Geometry: final body of the model. Coordinates: model frame, mm. A direction names the side the tool comes from. Give positions to 0.01 mm unless a question says otherwise; leave off trailing zeros. Write each loop counter-clockwise with the first axis right and the second up, starting at its lowest first coordinate (ties: lowest second). Pieces come first, ordered by that corner, then holes. Notation, with made-up numbers: (45.25, 65.5) - (65.25, 65.5) arc R33 cw to (65.25, 95.5) - close; hole circle Ø9 at (44.25, 45.5). An arc over 180 degrees is marked (long way). Return JSON: item names as keys, results as strings.
from build123d import *

# Parameters (mm, degrees)
SKETCH_1_W          = 126
SKETCH_1_H          = 28
EXTRUDE_1_DEPTH     = 5
FILLET_1_R          = 5
FILLET_2_R          = 0.5
SKETCH_3_R          = 1.5
CUT_EXTRUDE_1_DEPTH = 10
SKETCH_4_R          = 5
EXTRUDE_2_DEPTH     = 3
EXTRUDE_3_DEPTH     = 13
SKETCH_6_R          = 1.5
CUT_EXTRUDE_2_DEPTH = 6
SKETCH_7_R          = 13
EXTRUDE_4_DEPTH     = 33
SKETCH_8_R          = 5
EXTRUDE_5_DEPTH     = 3
SKETCH_9_R          = 13
EXTRUDE_6_DEPTH     = 1
SKETCH_10_R         = 1
EXTRUDE_7_DEPTH     = 4
SKETCH_11_R         = 9
EXTRUDE_8_DEPTH     = 4
SKETCH_12_W         = 6
SKETCH_12_H         = 1.146117225
EXTRUDE_9_DEPTH     = 8
SKETCH_13_W         = 13
SKETCH_13_H         = 5
EXTRUDE_10_DEPTH    = 3.9


with BuildPart() as part:
    # 草图1 → 凸台-拉伸1 (new, symmetric)
    with BuildSketch(Plane.XY):
        Rectangle(SKETCH_1_W, SKETCH_1_H)
    extrude(amount=EXTRUDE_1_DEPTH, both=True)

    # 圆角1
    fillet_1_edges = [part.edges().sort_by_distance(p)[0] for p in [
        (63, -14, 0),
        (-63, -14, 0),
        (-63, 14, 0),
        (63, 14, 0),
    ]]
    fillet(fillet_1_edges, radius=FILLET_1_R)

    # 圆角2
    fillet_2_edges = [part.edges().sort_by_distance(p)[0] for p in [
        (0, -14, -5),
        (0, -14, 5),
        (63, 0, -5),
        (-63, 0, -5),
        (0, 14, -5),
        (61.535533906, 12.535533906, -5),
        (61.535533906, -12.535533906, -5),
        (-61.535533906, 12.535533906, -5),
        (-61.535533906, -12.535533906, -5),
        (-63, 0, 5),
        (63, 0, 5),
        (0, 14, 5),
        (61.535533906, 12.535533906, 5),
        (61.535533906, -12.535533906, 5),
        (-61.535533906, 12.535533906, 5),
        (-61.535533906, -12.535533906, 5),
    ]]
    fillet(fillet_2_edges, radius=FILLET_2_R)

    # 草图3 → 切除-拉伸1 (cut)
    with BuildSketch(Plane.XZ.offset(14)):
        with Locations(Location((-40, 0, 0), (0, 0, 270))):
            Circle(SKETCH_3_R)
        with Locations(Location((40, 0, 0), (0, 0, 90))):
            Circle(SKETCH_3_R)
    cut_extrude_1 = extrude(amount=-CUT_EXTRUDE_1_DEPTH, mode=Mode.SUBTRACT)

    # 草图4 → 凸台-拉伸2 (add)
    with BuildSketch(Plane.XY.offset(5)):
        with Locations((47.75, 0)):
            Circle(SKETCH_4_R)
    extrude_2 = extrude(amount=EXTRUDE_2_DEPTH)

    # 草图5 → 凸台-拉伸3 (add)
    with BuildSketch(Plane.XY.offset(8)):
        Polygon((47.75, -3.75277675), (51, -1.876388375), (51, 1.876388375), (47.75, 3.75277675), (44.5, 1.876388375), (44.5, -1.876388375), align=None)
    extrude_3 = extrude(amount=EXTRUDE_3_DEPTH)

    # 草图6 → 切除-拉伸2 (cut)
    with BuildSketch(Plane.XY.offset(21)):
        with Locations((47.75, 0)):
            Circle(SKETCH_6_R)
    cut_extrude_2 = extrude(amount=-CUT_EXTRUDE_2_DEPTH, mode=Mode.SUBTRACT)

    # 镜向1: 凸台-拉伸2, 凸台-拉伸3, 切除-拉伸2 across plane
    add(extrude_2.mirror(Plane(origin=(0, 0, 0), x_dir=(0, 0, 1), z_dir=(1, 0, 0))))
    add(extrude_3.mirror(Plane(origin=(0, 0, 0), x_dir=(0, 0, 1), z_dir=(1, 0, 0))))
    add(cut_extrude_2.mirror(Plane(origin=(0, 0, 0), x_dir=(0, 0, 1), z_dir=(1, 0, 0))), mode=Mode.SUBTRACT)

    # 草图7 → 凸台-拉伸4 (add)
    with BuildSketch(Plane(origin=(0, 0, -5), x_dir=(-1, 0, 0), z_dir=(0, 0, -1))):
        with Locations(Location((0, 0, 0), (0, 0, 180))):
            Circle(SKETCH_7_R)
    extrude(amount=EXTRUDE_4_DEPTH)

    # 草图8 → 凸台-拉伸5 (add)
    with BuildSketch(Plane(origin=(0, 0, -38), x_dir=(-1, 0, 0), z_dir=(0, 0, -1))):
        Circle(SKETCH_8_R)
    extrude(amount=EXTRUDE_5_DEPTH)

    # 草图9 → 凸台-拉伸6 (add)
    with BuildSketch(Plane(origin=(0, 0, -41), x_dir=(-1, 0, 0), z_dir=(0, 0, -1))):
        with Locations(Location((0, 0, 0), (0, 0, 180))):
            Circle(SKETCH_9_R)
    extrude(amount=EXTRUDE_6_DEPTH)

    # 草图10 → 凸台-拉伸7 (add)
    with BuildSketch(Plane(origin=(0, 0, -42), x_dir=(-1, 0, 0), z_dir=(0, 0, -1))):
        Circle(SKETCH_10_R)
    extrude(amount=EXTRUDE_7_DEPTH)

    # 草图11 → 凸台-拉伸8 (add)
    with BuildSketch(Plane(origin=(0, 0, -46), x_dir=(-1, 0, 0), z_dir=(0, 0, -1))):
        Circle(SKETCH_11_R)
    extrude(amount=EXTRUDE_8_DEPTH)

    # 草图12 → 凸台-拉伸9 (add)
    with BuildSketch(Plane(origin=(0, 0, -42), x_dir=(-1, 0, 0), z_dir=(0, 0, -1))):
        with Locations((0, 9.822897289)):
            Rectangle(SKETCH_12_W, SKETCH_12_H)
    extrude(amount=EXTRUDE_9_DEPTH)

    # 草图13 → 凸台-拉伸10 (add)
    with BuildSketch(Plane(origin=(0, 0, -42), x_dir=(-1, 0, 0), z_dir=(0, 0, -1))):
        with Locations((0.124599067, -8.685467679)):
            Rectangle(SKETCH_13_W, SKETCH_13_H)
    extrude(amount=EXTRUDE_10_DEPTH)

    # 镜向2: 切除-拉伸1 across plane
    add(cut_extrude_1.mirror(Plane.ZX), mode=Mode.SUBTRACT)


solid = part.part
Q1. Section query A-A, the plane x = 30. Return the cut outline in (y, z), plus the area to 3 significant figures.
Answer key:
{"outline": "(-14, -4.5) arc R0.5 ccw to (-13.5, -5) - (13.5, -5) arc R0.5 ccw to (14, -4.5) - (14, 4.5) arc R0.5 ccw to (13.5, 5) - (-13.5, 5) arc R0.5 ccw to (-14, 4.5) - close", "area": "280 mm^2"}
Q2. Section query B-B, the plane z = 0. Return the cut outline in (x, y), plus the area to 3 significant figures.
Answer key:
{"outline": "(-63, -9) arc R5 ccw to (-58, -14) - (-41.5, -14) - (-41.5, -4) - (-38.5, -4) - (-38.5, -14) - (38.5, -14) - (38.5, -4) - (41.5, -4) - (41.5, -14) - (58, -14) arc R5 ccw to (63, -9) - (63, 9) arc R5 ccw to (58, 14) - (41.5, 14) - (41.5, 4) - (38.5, 4) - (38.5, 14) - (-38.5, 14) - (-38.5, 4) - (-41.5, 4) - (-41.5, 14) - (-58, 14) arc R5 ccw to (-63, 9) - close", "area": "3,390 mm^2"}
Q3. Section query C-C, the plane z = -30. Return the cut outline in (x, y), plus the area to 3 significant figures.
Answer key:
{"outline": "circle Ø26 at (0, 0)", "area": "531 mm^2"}
Q4. Pin query (flat end, axial travel): P1, Ø5, axis at x = -42, y = 11, coming from the -Z side; P2, Ø4, axis at y = 0, z = 12, coming from the -X side; P3, Ø4.5, axis at x = 0, z = -44, coming from the -Y side. Return the tip coordinate at first contact, or that it passes through.
Answer key:
{"P1": "stops at z = -5", "P2": "stops at x = -51", "P3": "stops at y = -13"}
Q5. Set-up query: faces 4 (the flat face through (-40, 4, 0)), 5 (the flat face through (0, 9.25, -46)), 6 (the flat face through (0, -11.185, -44)), 7 (the cylindrical face through (41.464, -9.07, -0.325)), 8 (the flat face through (0, -9.2, -45.9)). Return all of +Z, -Z, +X, -X, +Y, -Y with unobstructed straight access to the full face (end or side cutting, diameter ignored); none if empty.
Answer key:
{"face 4": "+Y", "face 5": "-Z, +X, -X", "face 6": "-Z, +X, -X, -Y", "face 7": "-Y", "face 8": "+X, -X, -Y"}
Q6. Material intervals for probe 1 along X at (y, z) = (-7.5, 0); probe 2 along Z at (x, y) = (-54.5, -6.25); probe 3 along Z at (x, y) = (40, 9.25), sorted ascending. Write a range as [from, to].
Answer key:
{"probe 1": "x = [-63, -41.5], [-38.5, 38.5], [41.5, 63]", "probe 2": "z = [-5, 5]", "probe 3": "z = [-5, -1.5], [1.5, 5]"}
Q7. Mould query, pull axis Y, two halves, no side actions, for faces 1 (the flat face through (-49.4, 2.8, 14.4)), 2 (the flat face through (6, 0, -41)), 3 (the flat face through (48, 0, 15)). Classes: pulls with the +Y half, pulls with the -Y half, needs draft (parallel to the pull), parting line crosses it, or undercut.
Answer key:
{"face 1": "pulls with the +Y half", "face 2": "needs draft", "face 3": "undercut"}
